Check sheet for the modelled part. Datum: model origin and axes. Units: mm. A direction names the side the tool comes from. Round coordinates to 2 decimals unless told otherwise and drop trailing zeros. Write each loop counter-clockwise with the first axis right and the second up, starting at its lowest first coordinate (ties: lowest second). Pieces come first, ordered by that corner, then holes. Notation, with made-up numbers: M -24.75,34.25 L -6.75,34.25 A36 cw -6.75,69.25 Z; hole C 3,54 d11. An arc over 180 degrees is marked long. One line per item, written item: value.
from build123d import *

# Parameters (mm, degrees)
SKETCH1_W             = 4.5
SKETCH1_H             = 30
BOSS_EXTRUDE1_DEPTH   = 4.5
SKETCH1_3_W           = 6
SKETCH1_3_H           = 30
BOSS_EXTRUDE2_DEPTH   = 37.5
SKETCH1_4_W           = 4.5
SKETCH1_4_H           = 30
BOSS_EXTRUDE3_DEPTH   = 7
CUT_EXTRUDE1_REACH    = 12.5
SKETCH2_R             = 7.5
CHAMFER1_SIZE         = 2
CHAMFER1_SIZE2        = 1.154700538
CHAMFER1_PART_2_SIZE  = 2
CHAMFER1_PART_2_SIZE2 = 1.154700538
CHAMFER1_PART_3_SIZE  = 2
CHAMFER1_PART_3_SIZE2 = 1.154700538


with BuildPart() as part:
    # Sketch1 → Boss-Extrude1 (new body)
    with BuildSketch(Plane(origin=(0, 0, 0), x_dir=(1, 0, 0), z_dir=(0, 1, 0))):
        with Locations((12.75, 15)):
            Rectangle(SKETCH1_W, SKETCH1_H)
    extrude(amount=BOSS_EXTRUDE1_DEPTH)

    # Sketch1<3> → Boss-Extrude2 (add)
    with BuildSketch(Plane(origin=(0, 0, 0), x_dir=(1, 0, 0), z_dir=(0, 1, 0))):
        with Locations((7.5, 15)):
            Rectangle(SKETCH1_3_W, SKETCH1_3_H)
    extrude(amount=BOSS_EXTRUDE2_DEPTH)

    # Sketch1<4> → Boss-Extrude3 (add)
    with BuildSketch(Plane(origin=(0, 0, 0), x_dir=(1, 0, 0), z_dir=(0, 1, 0))):
        with Locations((2.25, 15)):
            Rectangle(SKETCH1_4_W, SKETCH1_4_H)
    extrude(amount=BOSS_EXTRUDE3_DEPTH)

    # Sketch2 → Cut-Extrude1 (cut, up to next)
    with BuildSketch(Plane(origin=(10.5, 0, 0), x_dir=(0, 0, -1), z_dir=(1, 0, 0)), mode=Mode.PRIVATE) as cut_extrude1_sk1:
        with Locations((15, 22.5)):
            Circle(SKETCH2_R)
    cut_extrude1_tool1 = extrude(cut_extrude1_sk1.sketch, amount=-CUT_EXTRUDE1_REACH, mode=Mode.PRIVATE) & part.part
    add(cut_extrude1_tool1.solids().sort_by_distance((10.5, 22.5, -15))[0], mode=Mode.SUBTRACT)

    # Chamfer1
    chamfer1_edges = [part.edges().sort_by_distance(p)[0] for p in [
        (7.5, 37.5, -30),
    ]]
    chamfer1_side = [part.faces().sort_by_distance(p)[0] for p in [
        (7.5, 37.5, -15),
    ]]
    chamfer(chamfer1_edges, length=CHAMFER1_SIZE, length2=CHAMFER1_SIZE2, reference=chamfer1_side[0])

    # Chamfer1 part 2
    chamfer1_part_2_edges = [part.edges().sort_by_distance(p)[0] for p in [
        (7.5, 37.5, 0),
        (15, 2.25, 0),
    ]]
    chamfer1_part_2_side = [part.faces().sort_by_distance(p)[0] for p in [
        (7.286585366, 15.806910569, 0),
    ]]
    chamfer(chamfer1_part_2_edges, length=CHAMFER1_PART_2_SIZE, length2=CHAMFER1_PART_2_SIZE2, reference=chamfer1_part_2_side[0])

    # Chamfer1 part 3
    chamfer1_part_3_edges = [part.edges().sort_by_distance(p)[0] for p in [
        (15, 2.25, -30),
    ]]
    chamfer1_part_3_side = [part.faces().sort_by_distance(p)[0] for p in [
        (15, 2.25, -15),
    ]]
    chamfer(chamfer1_part_3_edges, length=CHAMFER1_PART_3_SIZE, length2=CHAMFER1_PART_3_SIZE2, reference=chamfer1_part_3_side[0])

    # Mirror1: part across plane


with BuildPart() as part_1:
    add(part.part)
    add(part.part.mirror(Plane(origin=(0, 7, 0), x_dir=(0, 0, 1), z_dir=(-1, 0, 0))))


solid = part_1.part
Q1. Draft check along Y on faces 4 (the flat face through (6, 14, -30)), 5 (the flat face through (7, 37.5, -15)), 6 (the cylindrical face through (-7.542, 29.936, -14.024)). Enter one of: pulls with the +Y half, pulls with the -Y half, needs draft (parallel to the pull), parting line crosses it, or undercut.
Completed:
face 4: needs draft
face 5: pulls with the +Y half
face 6: undercut
Q2. Access from +Z, -Z, +X, -X, +Y, -Y to the whole of each face (thin tool, end or side, straight path). Record for faces 1 (the flat face through (-4.5, 15, -11)), 2 (the flat face through (15, 2, -14)), 3 (the flat face through (-10.5, 13, -15)).
Completed:
face 1: +Z, -Z, +Y
face 2: +Z, -Z, +X, +Y, -Y
face 3: +Z, -Z, -X, +Y
Q3. Sectioned sample at B-B on y = 22.5. Enter the section's corners in (x, z), and give its area (3 significant figures).
Completed:
outline: M -10.5,-30 L -4.5,-30 L -4.5,-22.5 L -10.5,-22.5 Z; M -10.5,-7.5 L -4.5,-7.5 L -4.5,0 L -10.5,0 Z; M 4.5,-30 L 10.5,-30 L 10.5,-22.5 L 4.5,-22.5 Z; M 4.5,-7.5 L 10.5,-7.5 L 10.5,0 L 4.5,0 Z
area: 180 mm^2
Q4. Depth check by flat-ended pin: P1, Ø5, axis at y = 32.5, z = -17, coming from the +X side; P2, Ø1.4, axis at x = -12, z = -15, coming from the +Y side; P3, Ø15, axis at y = 17.5, z = -9.5, coming from the -X side; P4, Ø12, axis at y = 22.5, z = -15, coming from the -X side. Enter the tip coordinate at first touch or a pass-through.
Completed:
P1: x = 10.5
P2: y = 4.5
P3: x = -10.5
P4: through
Q5. Sectioned sample at C-C on x = -8. Enter the section's corners in (y, z), and give its area (3 significant figures).
Completed:
outline: M 0,-30 L 36.35,-30 L 37.5,-28 L 37.5,-1.15 L 35.5,0 L 0,0 Z; hole C 22.5,-15 d15
area: 946 mm^2
Q6. Sectioned sample at D-D on y = 10. Enter the section's corners in (x, z).
Completed:
outline: M -10.5,-30 L -4.5,-30 L -4.5,0 L -10.5,0 Z; M 4.5,-30 L 10.5,-30 L 10.5,0 L 4.5,0 Z
Q7. Scan lines: line 1 (X direction, y = 19, z = -2); line 2 (Y direction, x = 6.05, z = -15); line 3 (Y direction, x = -4, z = -4). Record each from-to range of solid material in increasing order. Write a range as [from, to].
Completed:
line 1: [-10.5, -4.5], [4.5, 10.5]
line 2: [0, 15], [30, 37.5]
line 3: [0, 7]
Q8. Sectioned sample at A-A on z = -15. Enter the section's corners in (x, y), and give its area (4 significant figures).
Completed:
outline: M -15,0 L 15,0 L 15,4.5 L 10.5,4.5 L 10.5,15 L 4.5,15 L 4.5,7 L -4.5,7 L -4.5,15 L -10.5,15 L -10.5,4.5 L -15,4.5 Z; M -10.5,30 L -4.5,30 L -4.5,37.5 L -10.5,37.5 Z; M 4.5,30 L 10.5,30 L 10.5,37.5 L 4.5,37.5 Z
area: 373.5 mm^2
